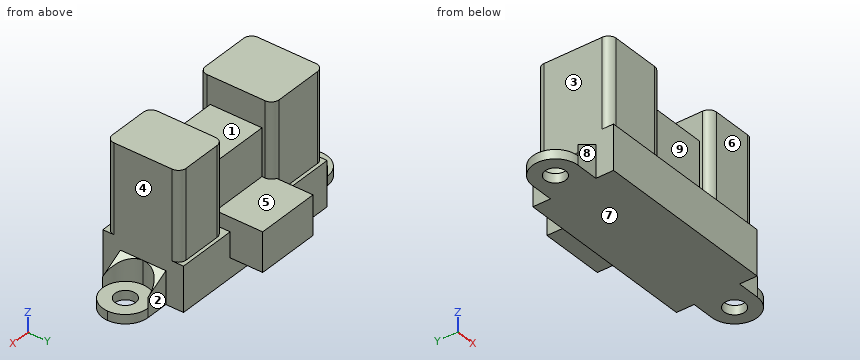
from build123d import *

# Parameters (mm, degrees)
F0_R      = 1.6764
F1_DEPTH  = 1.4732
F3_DEPTH  = 3.81
F5_DEPTH  = 7.366
F7_DEPTH  = 7.239
F9_DEPTH  = 14.351
F10_W     = 10.287
F10_H     = 8.382
F11_DEPTH = 9.906
F12_W     = 10.414
F12_H     = 6.35
F13_DEPTH = 7.62


with BuildPart() as f1:
    # F0 (on Top) → F1 (new body)
    with BuildSketch(Plane.XY):
        Polygon((14.859, 3.683), (14.859, 6.5405), (-14.859, 6.5405), (-14.859, 3.683), (-14.859, 0), (-14.859, -3.683), (-14.859, -6.5405), (14.859, -6.5405), (14.859, -3.683), (14.859, 0), align=None)
        with BuildLine():
            Line((18.542, 3.683), (14.859, 3.683))
            Line((14.859, 3.683), (14.859, 0))
            ThreePointArc((14.859, 0), (15.937726, 2.604274), (18.542, 3.683))
        make_face()
        with BuildLine():
            Line((-14.859, 0), (-14.859, 3.683))
            Line((-14.859, 3.683), (-18.542, 3.683))
            ThreePointArc((-18.542, 3.683), (-15.937726, 2.604274), (-14.859, 0))
        make_face()
        with BuildLine():
            ThreePointArc((18.542, -3.683), (15.937726, -2.604274), (14.859, 0))
            Line((14.859, 0), (14.859, -3.683))
            Line((14.859, -3.683), (18.542, -3.683))
        make_face()
        with BuildLine():
            ThreePointArc((18.542, 3.683), (15.937726, 2.604274), (14.859, 0))
            ThreePointArc((14.859, 0), (15.937726, -2.604274), (18.542, -3.683))
            ThreePointArc((18.542, -3.683), (21.146274, -2.604274), (22.225, 0))
            ThreePointArc((22.225, 0), (21.146274, 2.604274), (18.542, 3.683))
        make_face()
        with Locations((18.542, 0)):
            Circle(F0_R, mode=Mode.SUBTRACT)
        with BuildLine():
            ThreePointArc((-18.542, -3.683), (-15.937726, -2.604274), (-14.859, 0))
            ThreePointArc((-14.859, 0), (-15.937726, 2.604274), (-18.542, 3.683))
            ThreePointArc((-18.542, 3.683), (-22.225, 0), (-18.542, -3.683))
        make_face()
        with Locations((-18.542, 0)):
            Circle(F0_R, mode=Mode.SUBTRACT)
        with BuildLine():
            Line((-14.859, -3.683), (-14.859, 0))
            ThreePointArc((-14.859, 0), (-15.937726, -2.604274), (-18.542, -3.683))
            Line((-18.542, -3.683), (-14.859, -3.683))
        make_face()
    extrude(amount=F1_DEPTH)



with BuildPart() as f3:
    # F2 (on face) → F3 (new body)
    with BuildSketch(Plane.XY.offset(1.4732)):
        with BuildLine():
            Line((-14.859, 3.683), (-18.542, 3.683))
            ThreePointArc((-18.542, 3.683), (-15.937726, 2.604274), (-14.859, 0))
            Line((-14.859, 0), (-14.859, 3.683))
        make_face()
        with BuildLine():
            Line((-14.859, -3.683), (-14.859, 0))
            ThreePointArc((-14.859, 0), (-15.937726, -2.604274), (-18.542, -3.683))
            Line((-18.542, -3.683), (-14.859, -3.683))
        make_face()
        with BuildLine():
            Line((14.859, -3.683), (18.542, -3.683))
            ThreePointArc((18.542, -3.683), (15.937726, -2.604274), (14.859, 0))
            Line((14.859, 0), (14.859, -3.683))
        make_face()
        with BuildLine():
            Line((14.859, 3.683), (14.859, 0))
            ThreePointArc((14.859, 0), (15.937726, 2.604274), (18.542, 3.683))
            Line((18.542, 3.683), (14.859, 3.683))
        make_face()
    extrude(amount=F3_DEPTH)

    # F4 (on face) → F5 (cut, through all)
    with BuildSketch(Plane.XZ.offset(3.683)):
        Polygon((-18.542, 5.2832), (-18.542, 3.2004), (-14.859, 5.2832), align=None)
        Polygon((14.859, 5.2832), (18.542, 3.2004), (18.542, 5.2832), align=None)
    extrude(amount=-F5_DEPTH, mode=Mode.SUBTRACT)


with BuildPart() as f1_1:
    add(f1.part)

    add(f3.part)  # F7 merges F3
    # F6 (on Top) → F7 (join)
    with BuildSketch(Plane.XY):
        Polygon((14.859, 3.683), (14.859, 6.5405), (-14.859, 6.5405), (-14.859, 3.683), (-14.859, 0), (-14.859, -3.683), (-14.859, -6.5405), (14.859, -6.5405), (14.859, -3.683), (14.859, 0), align=None)
    extrude(amount=F7_DEPTH)

    # F8 (on face) → F9 (join)
    with BuildSketch(Plane.XY.offset(7.239)):
        with BuildLine():
            ThreePointArc((-4.3688, 4.7117), (-4.740774, 5.609726), (-5.6388, 5.9817))
            Line((-5.6388, 5.9817), (-13.589, 5.9817))
            ThreePointArc((-13.589, 5.9817), (-14.487026, 5.609726), (-14.859, 4.7117))
            Line((-14.859, 4.7117), (-14.859, -4.7117))
            ThreePointArc((-14.859, -4.7117), (-14.487026, -5.609726), (-13.589, -5.9817))
            Line((-13.589, -5.9817), (-5.6388, -5.9817))
            ThreePointArc((-5.6388, -5.9817), (-4.740774, -5.609726), (-4.3688, -4.7117))
            Line((-4.3688, -4.7117), (-4.3688, 4.7117))
        make_face()
        with BuildLine():
            ThreePointArc((14.859, 4.7117), (14.487026, 5.609726), (13.589, 5.9817))
            Line((13.589, 5.9817), (7.1882, 5.9817))
            ThreePointArc((7.1882, 5.9817), (6.290174, 5.609726), (5.9182, 4.7117))
            Line((5.9182, 4.7117), (5.9182, -4.7117))
            ThreePointArc((5.9182, -4.7117), (6.290174, -5.609726), (7.1882, -5.9817))
            Line((7.1882, -5.9817), (13.589, -5.9817))
            ThreePointArc((13.589, -5.9817), (14.487026, -5.609726), (14.859, -4.7117))
            Line((14.859, -4.7117), (14.859, 4.7117))
        make_face()
    extrude(amount=F9_DEPTH)

    # F10 (on face) → F11 (join)
    with BuildSketch(Plane.XY.offset(7.239)):
        with Locations((0.7747, 0)):
            Rectangle(F10_W, F10_H)
    extrude(amount=F11_DEPTH)

    # F12 (on face) → F13 (join)
    with BuildSketch(Plane(origin=(0, 4.191, 0), x_dir=(-1, 0, 0), z_dir=(0, 1, 0))):
        with Locations((0, 6.35)):
            Rectangle(F12_W, F12_H)
    extrude(amount=F13_DEPTH)


solid = f1_1.part
Input: part model. Units: mm. Frame: model coordinates. Face numbers are marked on the shaded views. A direction names the side the tool comes from. Give positions to 0.01 mm unless a question says otherwise; leave off trailing zeros. Order: outer loops, then holes, each group sorted by start corner. A loop starts at its lowest first (then second) coordinate and runs counter-clockwise, first axis right, second up. Notation, with made-up numbers: (-14, 68.25) -> (-2, 68.25) arc R14 cw to (-2, 73.25) -> close; hole circle Ø4 at (-7, 27). An arc over 180 degrees is marked (long way). Use one line per item in the form item = value.
1) Line query: probe 1 along X at (y, z) = (-4.25, 18); probe 2 along X at (y, z) = (-1, 1); probe 3 along X at (y, z) = (2.5, 8.25). Output: solid intervals per line, ascending.
Response values:
probe_1 = -14.86 to -4.37, 5.92 to 14.86
probe_2 = -22.09 to -19.89, -17.2 to 17.2, 19.89 to 22.09
probe_3 = -14.86 to 14.86
2) Reachability of the marked faces 5, 6, 7, 8 and 9 from +Z, -Z, +X, -X, +Y, -Y: full face, straight path, thin tool, end or side. Return the list, or none.
Response values:
face_5 = +Z, +Y
face_6 = +Z, +X, -X, -Y
face_7 = -Z, +X, -X, +Y, -Y
face_8 = +Z, -Z, -X, -Y
face_9 = +Z, -Y
3) Section D-D, the plane x = -7.5. Return loops of the section in (y, z), and give its area (3 significant figures).
Response values:
outline = (-6.54, 0) -> (6.54, 0) -> (6.54, 7.24) -> (5.98, 7.24) -> (5.98, 21.59) -> (-5.98, 21.59) -> (-5.98, 7.24) -> (-6.54, 7.24) -> close
area = 266 mm^2
4) Section B-B, the plane z = 2.75. Return loops of the section in (x, y), and give its area (3 significant figures).
Response values:
outline = (-18.54, -3.68) -> (-14.86, -3.68) -> (-14.86, -6.54) -> (14.86, -6.54) -> (14.86, -3.68) -> (18.54, -3.68) arc R3.68 cw to (14.86, 0) arc R3.68 cw to (18.54, 3.68) -> (14.86, 3.68) -> (14.86, 6.54) -> (-14.86, 6.54) -> (-14.86, 3.68) -> (-18.54, 3.68) arc R3.68 cw to (-14.86, 0) arc R3.68 cw to start
area = 400 mm^2
5) Section A-A, the plane x = 1. Return loops of the section in (y, z) (1 decimal), and give its area (3 significant figures).
Response values:
outline = (-6.5, 0) -> (6.5, 0) -> (6.5, 3.2) -> (11.8, 3.2) -> (11.8, 9.5) -> (4.2, 9.5) -> (4.2, 17.1) -> (-4.2, 17.1) -> (-4.2, 7.2) -> (-6.5, 7.2) -> close
area = 217 mm^2
6) Section C-C, the plane y = 1. Return loops of the section in (x, z) (3 decimals), and give its area (3 significant figures).
Response values:
outline = (-22.087, 0) -> (-19.887, 0) -> (-19.887, 1.473) -> (-22.087, 1.473) -> close; (-17.197, 0) -> (17.197, 0) -> (17.197, 1.473) -> (14.997, 1.473) -> (14.997, 5.205) -> (14.859, 5.283) -> (14.859, 21.59) -> (5.918, 21.59) -> (5.918, 17.145) -> (-4.369, 17.145) -> (-4.369, 21.59) -> (-14.859, 21.59) -> (-14.859, 5.283) -> (-14.997, 5.205) -> (-14.997, 1.473) -> (-17.197, 1.473) -> close; (19.887, 0) -> (22.087, 0) -> (22.087, 1.473) -> (19.887, 1.473) -> close
area = 610 mm^2
7) Mould query, pull axis X, two halves, no side actions, for the marked faces 1, 2, 3 and 4. Classes: pulls with the +X half, pulls with the -X half, needs draft (parallel to the pull), parting line crosses it, or undercut.
Response values:
face_1 = undercut
face_2 = needs draft
face_3 = pulls with the -X half
face_4 = pulls with the +X half
8) First-contact query: pin 1 Ø2.5 at (x, z) = (-10.5, 14.5) entering from -Y; pin 2 Ø1.5 at (x, z) = (-7, 3) entering from +Y; pin 3 Ø12 at (x, z) = (7, 16.5) entering from +Y; pin 4 Ø3 at (x, z) = (1, 10.5) entering from +Y. Flat tips, straight axial feed; report the tip coordinate or a pass-through.
Response values:
pin_1 = -5.98
pin_2 = 6.54
pin_3 = 5.98
pin_4 = 11.81
